Read the model definition and answer for the solid it produces. Units are mm, in the model's axes. Give positions to 0.01 mm unless a question says otherwise; leave off trailing zeros. Order: outer loops, then holes, each group sorted by start corner. A loop starts at its lowest first (then second) coordinate and runs counter-clockwise, first axis right, second up. Notation, with made-up numbers: M 22.25,-12.75 L 31.25,-12.75 A17 cw 31.25,-5.75 Z; hole C -27.75,35.5 d1. An arc over 180 degrees is marked long. One line per item, written item: value. Start each with the question number.
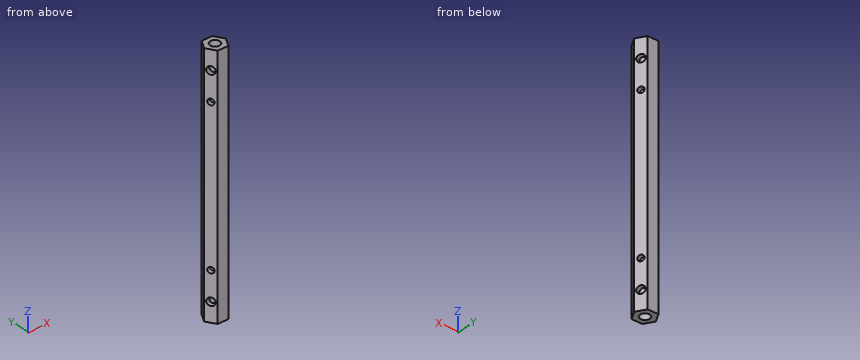
from build123d import *

# Parameters (mm, degrees)
SKETCH1_R           = 3.2639
BOSS_EXTRUDE1_DEPTH = 165.1
SKETCH2_R           = 2.0193
SKETCH2_R_2         = 2.6289
CUT_EXTRUDE1_DEPTH  = 16.875


with BuildPart() as part:
    # Sketch1 → Boss-Extrude1 (new body)
    with BuildSketch(Plane.XY):
        Polygon((-3.666174209, 6.35), (-7.332348419, 0), (-3.666174209, -6.35), (3.666174209, -6.35), (7.332348419, 0), (3.666174209, 6.35), align=None)
        Circle(SKETCH1_R, mode=Mode.SUBTRACT)
    extrude(amount=BOSS_EXTRUDE1_DEPTH)

    # Sketch2 → Cut-Extrude1 (cut, through all)
    with BuildSketch(Plane(origin=(5.499261314, 3.175, 0), x_dir=(0, 0, -1), z_dir=(0.866025404, 0.5, 0))):
        with Locations((-31.75, 0)):
            Circle(SKETCH2_R)
        with Locations((-133.35, 0)):
            Circle(SKETCH2_R)
        with Locations((-12.7, 0)):
            Circle(SKETCH2_R_2)
        with Locations((-152.4, 0)):
            Circle(SKETCH2_R_2)
    extrude(amount=-CUT_EXTRUDE1_DEPTH, mode=Mode.SUBTRACT)


solid = part.part
Q1. Consider probe 1 along X at (y, z) = (0, 104); probe 2 along Y at (x, z) = (0, 146); probe 3 along Z at (x, y) = (3, 3). Determine where each line is inside the solid, lowest interval first.
Q2. Each of these flat-tipped pins is pushed along its axis until it touches: pin 1 (1 mm diameter, centred on x = -5.5, z = 139.5, fed in from +Y); pin 2 (5 mm diameter, centred on y = 3, z = 39, fed in from -X). Where does it stop, or does it pass through?
Q3. Find section A-A, the plane z = 23. Give the vertices of the cut face in (x, y).
Evaluation:
1. probe 1: -7.33 to -3.26, 3.26 to 7.33
1. probe 2: -6.35 to -3.26, 3.26 to 6.35
1. probe 3: 0 to 10.31, 15.09 to 30.06, 33.44 to 131.66, 135.04 to 150.01, 154.79 to 165.1
2. pin 1: y = 4.04
2. pin 2: x = -7.04
3. outline: M -7.33,0 L -3.67,-6.35 L 3.67,-6.35 L 7.33,0 L 3.67,6.35 L -3.67,6.35 Z; hole C 0,0 d6.53
